Here's how the part is built. I have some questions about the finished solid (model axes, mm). Coordinates: 2 decimals unless noted, no trailing zeros. Write each loop counter-clockwise with the first axis right and the second up, starting at its lowest first coordinate (ties: lowest second). Pieces come first, ordered by that corner, then holes.
from build123d import *

# Parameters (mm, degrees)
CYLINDER144_R     = 0.8
CYLINDER144_DEPTH = 10
CYLINDER136_R     = 0.2
CYLINDER136_DEPTH = 9
CYLINDER_R        = 1.1
CYLINDER_DEPTH    = 4
CYLINDER139_R     = 1.1
CYLINDER139_DEPTH = 4
CYLINDER138_R     = 0.165
CYLINDER138_DEPTH = 8
CYLINDER143_R     = 0.8
CYLINDER143_DEPTH = 10
CYLINDER142_R     = 2.5
CYLINDER142_DEPTH = 1.8
CYLINDER141_R     = 2.5
CYLINDER141_DEPTH = 1.8
CYLINDER140_R     = 0.35
CYLINDER140_DEPTH = 1
BOX_W             = 100
BOX_H             = 0.75
BOX_DEPTH         = 0.6


with BuildPart() as cylinder001:
    # Cylinder144 → Cylinder144 (new body)
    with BuildSketch(Plane(origin=(6.3, -2.8, -1), x_dir=(1, 0, 0), z_dir=(0, 0, 1))):
        Circle(CYLINDER144_R)
    extrude(amount=CYLINDER144_DEPTH)


with BuildPart() as bowtienozzle:
    # Cylinder136 → Cylinder136 (new body)
    with BuildSketch(Plane.XY):
        Circle(CYLINDER136_R)
    extrude(amount=CYLINDER136_DEPTH)


with BuildPart() as mountinghole1:
    # Cylinder → Cylinder (new body)
    with BuildSketch(Plane(origin=(-50, 0, -1), x_dir=(1, 0, 0), z_dir=(0, 0, 1))):
        Circle(CYLINDER_R)
    extrude(amount=CYLINDER_DEPTH)


with BuildPart() as mountinghole2:
    # Cylinder139 → Cylinder139 (new body)
    with BuildSketch(Plane(origin=(50, 0, -1), x_dir=(1, 0, 0), z_dir=(0, 0, 1))):
        Circle(CYLINDER139_R)
    extrude(amount=CYLINDER139_DEPTH)


with BuildPart() as fusion001:
    # Cylinder138 → Cylinder138 (new body)
    with BuildSketch(Plane(origin=(0, 0, 0), x_dir=(1, 0, 0), z_dir=(0, 1, 0))):
        Circle(CYLINDER138_R)
    extrude(amount=CYLINDER138_DEPTH)

    # Fusion001: union BowTieNozzle, MountingHole1, MountingHole2
    add(bowtienozzle.part)
    add(mountinghole1.part)
    add(mountinghole2.part)


with BuildPart() as fusion003:
    # Cylinder143 → Cylinder143 (new body)
    with BuildSketch(Plane(origin=(-6.3, -2.8, -1), x_dir=(1, 0, 0), z_dir=(0, 0, 1))):
        Circle(CYLINDER143_R)
    extrude(amount=CYLINDER143_DEPTH)

    # Fusion003: union Cylinder001, Fusion001
    add(cylinder001.part)
    add(fusion001.part)


with BuildPart() as obj1:
    # Cylinder142 → Cylinder142 (new body)
    with BuildSketch(Plane(origin=(50, 0, -0.3), x_dir=(1, 0, 0), z_dir=(0, 0, 1))):
        Circle(CYLINDER142_R)
    extrude(amount=CYLINDER142_DEPTH)


with BuildPart() as obj2:
    # Cylinder141 → Cylinder141 (new body)
    with BuildSketch(Plane(origin=(-50, 0, -0.3), x_dir=(1, 0, 0), z_dir=(0, 0, 1))):
        Circle(CYLINDER141_R)
    extrude(amount=CYLINDER141_DEPTH)


with BuildPart() as nozzle_od:
    # Cylinder140 → Cylinder140 (new body)
    with BuildSketch(Plane.XY.offset(0.3)):
        Circle(CYLINDER140_R)
    extrude(amount=CYLINDER140_DEPTH)


with BuildPart() as cut004:
    # Box → Box (new body)
    with BuildSketch(Plane(origin=(-50, -0.375, -0.3), x_dir=(1, 0, 0), z_dir=(0, 0, 1))):
        with Locations((50, 0.375)):
            Rectangle(BOX_W, BOX_H)
    extrude(amount=BOX_DEPTH)

    # Fusion: union obj1, obj2, Nozzle_OD
    add(obj1.part)
    add(obj2.part)
    add(nozzle_od.part)

    # Cut004: cut Fusion003
    add(fusion003.part, mode=Mode.SUBTRACT)


with BuildPart() as cut004_1:
    # Cut004 placement: moved
    add(cut004.part.moved(Location((0, 10, 0))))


solid = cut004_1.part
1. I want a section at C-C (x = -16.5). List the corners of the cut face in (y, z) for me (3 decimals).
2. I want a section at B-B (z = 0.65). List the corners of the cut face in (x, y) for me.
3. Thinking about a two-plate mould opening in X: for faces 1 (the face through (49.13, 9.33, 0.59)), 2 (the face through (-49, 9, 1.5)), which applies, pulls with the +X half, pulls with the -X half, needs draft (parallel to the pull), parting line crosses it, or undercut?
4. I want a section at A-A (x = 50). List the corners of the cut face in (y, z) for me.
5. If I drill on line 1 (X direction, y = 10, z = 0.15); line 2 (Y direction, x = 50, z = 0.5); line 3 (Y direction, x = 17.5, z = -0.1) (3 decimals), over which ranges is the centre line in solid material (lowest first)?
6. For pin 1 Ø0.7 at (x, z) = (14.5, 0) entering from -Y (3 decimals); pin 2 Ø0.8 at (x, y) = (10, 10) entering from +Z; pin 3 Ø0.8 at (x, y) = (0, 10) entering from +Z, each with a flat end and sliding along its axis, tell me the tip position at first contact or that it passes through.
Response values:
1. outline: (9.625, -0.3) - (10.375, -0.3) - (10.375, 0.3) - (9.625, 0.3) - close
2. outline: circle Ø5 at (-50, 10); circle Ø0.7 at (0, 10); circle Ø5 at (50, 10); hole circle Ø2.2 at (-50, 10); hole circle Ø0.4 at (0, 10); hole circle Ø2.2 at (50, 10)
3. face 1: undercut
3. face 2: needs draft
4. outline: (7.5, -0.3) - (8.9, -0.3) - (8.9, 1.5) - (7.5, 1.5) - close; (11.1, -0.3) - (12.5, -0.3) - (12.5, 1.5) - (11.1, 1.5) - close
5. line 1: x = -52.5 to -51.1, -48.9 to -0.2, 0.2 to 48.9, 51.1 to 52.5
5. line 2: y = 7.5 to 8.9, 11.1 to 12.5
5. line 3: y = 9.625 to 10.375
6. pin 1: stops at y = 9.625
6. pin 2: stops at z = 0.3
6. pin 3: stops at z = 1.3
